Work out the finished part from the listing and answer in its coordinate system (mm). Face numbers are marked on the shaded views. A direction names the side the tool comes from. Coordinates: 2 decimals unless noted, no trailing zeros. Loops run counter-clockwise (first coordinate to the right, second up) from the corner with the lowest first, then second, coordinate; pieces in that order, holes last. Notation, with made-up numbers: (-5.5, 22) -> (39.5, 22) arc R21 cw to (39.5, 48) -> close; hole circle Ø10 at (21, 89.5). An arc over 180 degrees is marked (long way). Use a Markdown table: item, result.
Autodesk Inventor part; units mm, degrees
ref_plane "YZ Plane" through (0, 0, 0) normal (1, 0, 0) x (0, 1, 0)
ref_plane "XZ Plane" through (0, 0, 0) normal (0, 1, 0) x (-1, 0, 0)
ref_plane "XY Plane" through (0, 0, 0) normal (0, 0, 1) x (1, 0, 0)
sketch "Sketch1" plane through (0, 0, 0) normal (0, 0, 1) x (1, 0, 0)
  circle A0 centre (0, 0) radius 5
  dimension "d0" = 10
extrude "Extrusion1" add sketch "Sketch1" along normal blind 14.75
sketch "Sketch2" plane through (0, 0, 14.75) normal (0, 0, 1) x (1, 0, 0)
  circle A0 centre (0, 0) radius 1.6
  dimension "d3" = 3.2
extrude "Extrusion2" cut sketch "Sketch2" against normal blind 14.75
sketch "Sketch3" plane through (0, 0, 14.75) normal (0, 0, 1) x (1, 0, 0)
  line L0 (0, 3.4641) -> (3, 1.7321)
  line L1 (3, 1.7321) -> (3, -1.7321)
  line L2 (3, -1.7321) -> (0, -3.4641)
  line L3 (0, -3.4641) -> (-3, -1.7321)
  line L4 (-3, -1.7321) -> (-3, 1.7321)
  line L5 (-3, 1.7321) -> (0, 3.4641)
  point P0 (0, 0)
  point P1 (0, 0)
  dimension "d6" = 6
extrude "Extrusion3" cut sketch "Sketch3" against normal blind 3
sketch "Sketch4" plane through (0, 0, 0) normal (0, 0, -1) x (-1, 0, 0)
  circle A0 centre (0, 0) radius 1.6
  line L0 (0, 3.4641) -> (-3, 1.7321)
  line L1 (3, 1.7321) -> (0, 3.4641)
  line L2 (3, -1.7321) -> (3, 1.7321)
  line L3 (0, -3.4641) -> (3, -1.7321)
  line L4 (-3, -1.7321) -> (0, -3.4641)
  line L5 (-3, 1.7321) -> (-3, -1.7321)
extrude "Extrusion4" cut sketch "Sketch4" against normal blind 3
properties part number "post"
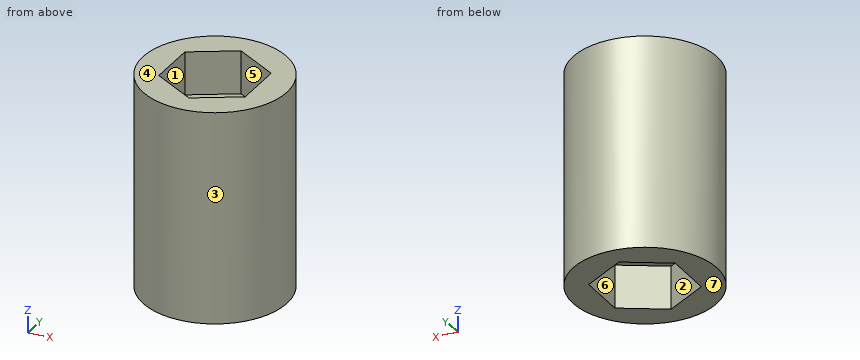
Q1. Section C-C on x = -0.75 is taken. Determine the outline of the cut face in (y, z).
Solved:
| item | result |
|---|---|
| outline | (-4.94, 0) -> (-3.03, 0) -> (-3.03, 3) -> (-1.41, 3) -> (-1.41, 11.75) -> (-3.03, 11.75) -> (-3.03, 14.75) -> (-4.94, 14.75) -> close; (1.41, 3) -> (3.03, 3) -> (3.03, 0) -> (4.94, 0) -> (4.94, 14.75) -> (3.03, 14.75) -> (3.03, 11.75) -> (1.41, 11.75) -> close |
Q2. Section D-D on y = 3 is taken. Determine the outline of the cut face in (x, z).
Solved:
| item | result |
|---|---|
| outline | (-4, 0) -> (-0.8, 0) -> (-0.8, 3) -> (0.8, 3) -> (0.8, 0) -> (4, 0) -> (4, 14.75) -> (0.8, 14.75) -> (0.8, 11.75) -> (-0.8, 11.75) -> (-0.8, 14.75) -> (-4, 14.75) -> close |
Q3. For the marked faces 5, 6 and 7, determine the directions among +Z, -Z, +X, -X, +Y, -Y from which every point of the face is accessible in a straight line to the end or side of a thin tool.
Solved:
| item | result |
|---|---|
| face 5 | +Z |
| face 6 | -Z |
| face 7 | -Z, +X, -X, +Y, -Y |
Q4. Section B-B on z = 2.5 is taken. Determine the outline of the cut face in (x, y), and give its area (3 significant figures).
Solved:
| item | result |
|---|---|
| outline | circle Ø10 at (0, 0); hole (-3, -1.73) -> (0, -3.46) -> (3, -1.73) -> (3, 1.73) -> (0, 3.46) -> (-3, 1.73) -> close |
| area | 47.4 mm² |
Q5. Determine the mould class of the marked faces 1, 2, 3 and 4 for opening direction X: pulls with the +X half, pulls with the -X half, needs draft (parallel to the pull), parting line crosses it, or undercut.
Solved:
| item | result |
|---|---|
| face 1 | undercut |
| face 2 | undercut |
| face 3 | parting line crosses it |
| face 4 | needs draft |
Q6. Given pin 1 Ø2 at (x, z) = (0.5, 2.5) entering from +Y; pin 2 Ø3 at (y, z) = (-3.5, 4.5) entering from -X; pin 3 Ø1.5 at (y, z) = (3.5, 7) entering from +X; pin 4 Ø3 at (x, y) = (0, 0) entering from +Z, each flat-ended and moving along its own axis, determine where each tip first touches the part or whether it passes through.
Solved:
| item | result |
|---|---|
| pin 1 | y = 5 |
| pin 2 | x = -4.58 |
| pin 3 | x = 4.18 |
| pin 4 | through |
Q7. Section A-A on y = 0 is taken. Determine the outline of the cut face in (x, z).
Solved:
| item | result |
|---|---|
| outline | (-5, 0) -> (-3, 0) -> (-3, 3) -> (-1.6, 3) -> (-1.6, 11.75) -> (-3, 11.75) -> (-3, 14.75) -> (-5, 14.75) -> close; (1.6, 3) -> (3, 3) -> (3, 0) -> (5, 0) -> (5, 14.75) -> (3, 14.75) -> (3, 11.75) -> (1.6, 11.75) -> close |
Q8. Consider line 1 (Y direction, x = 0, z = 9.5); line 2 (X direction, y = 2.25, z = 13); line 3 (X direction, y = 3.25, z = 12.25). Determine where each line is inside the solid, lowest interval first. Write a range as [from, to].
Solved:
| item | result |
|---|---|
| line 1 | [-5, -1.6], [1.6, 5] |
| line 2 | [-4.47, -2.1], [2.1, 4.47] |
| line 3 | [-3.8, -0.37], [0.37, 3.8] |
